Geometry: see drawing. Coordinates: mm, zero at the bounding-box minimum. A direction names the side the tool comes from. Give positions to 0.01 mm unless a question says otherwise; leave off trailing zeros. Loops run counter-clockwise (first coordinate to the right, second up) from the corner with the lowest first, then second, coordinate; pieces in that order, holes last. Notation, with made-up numbers: M -20.5,88.25 L -10.5,88.25 A16 ccw -10.5,113.25 Z; hole C 30,57 d5. An arc over 180 degrees is marked long. Put each result on its own line as item: value.
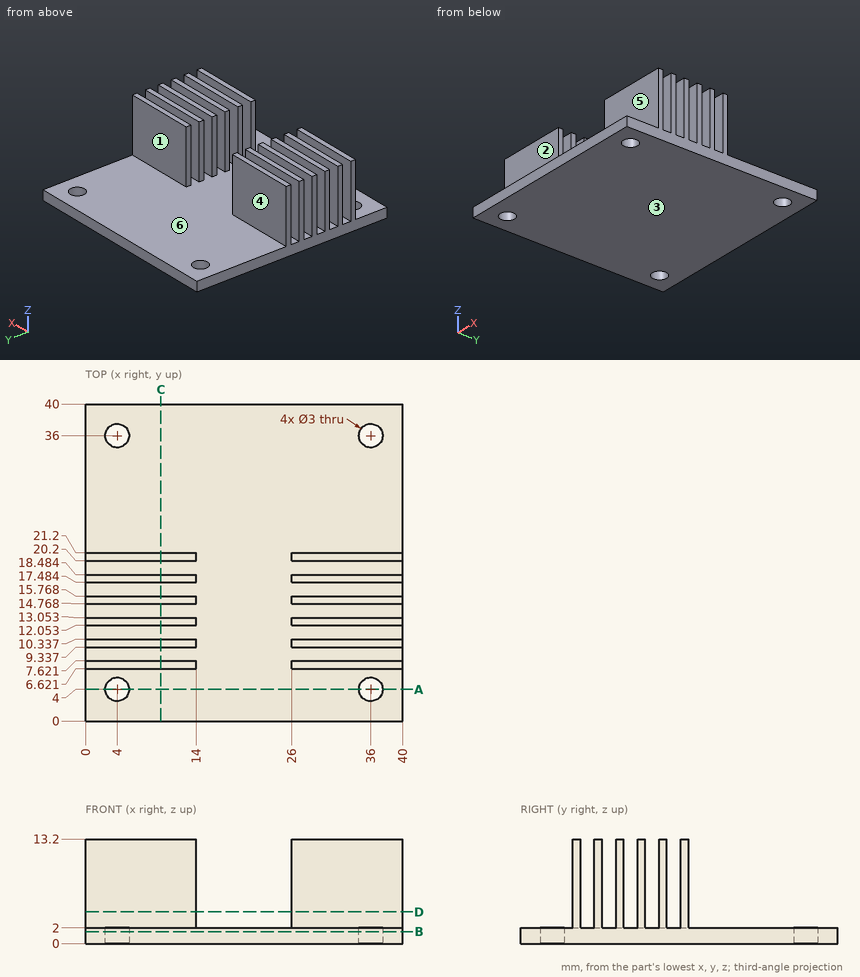
Item 1: Line query: probe 1 along Y at (x, z) = (7.5, 3.25) (1 decimal); probe 2 along Y at (x, z) = (36, 1.55); probe 3 along X at (y, z) = (12.5, 11.75). Output: solid intervals per line, ascending. Write a range as [from, to].
Output values:
probe 1: [6.6, 7.6], [9.3, 10.3], [12.1, 13.1], [14.8, 15.8], [17.5, 18.5], [20.2, 21.2]
probe 2: [0, 2.5], [5.5, 34.5], [37.5, 40]
probe 3: [0, 14], [26, 40]
Item 2: Section B-B on z = 1.5. Output: boundary loops of the cut face in (x, y).
Output values:
outline: M 0,0 L 40,0 L 40,40 L 0,40 Z; hole C 4,4 d3; hole C 4,36 d3; hole C 36,4 d3; hole C 36,36 d3
Item 3: Set-up query: the marked faces 1, 2 and 3. Return all of +Z, -Z, +X, -X, +Y, -Y with unobstructed straight access to the full face (end or side cutting, diameter ignored); none if empty.
Output values:
face 1: +Z, +X, -X, +Y
face 2: +Z, +X, -X, -Y
face 3: -Z, +X, -X, +Y, -Y
Item 4: Section A-A on y = 4. Output: boundary loops of the cut face in (x, z).
Output values:
outline: M 0,0 L 2.5,0 L 2.5,2 L 0,2 Z; M 5.5,0 L 34.5,0 L 34.5,2 L 5.5,2 Z; M 37.5,0 L 40,0 L 40,2 L 37.5,2 Z
Item 5: Section D-D on z = 4. Count the separate pieces of the cut face and the enclosed holes in it, then the cut area to 3 significant figures.
Output values:
separate pieces: 12
enclosed holes: 0
area: 168 mm²
Item 6: Pin query (flat end, axial travel): pin 1 Ø5.5 at (x, z) = (30.5, 10.5) entering from +Y; pin 2 Ø5.5 at (x, z) = (34.5, 9) entering from -Y; pin 3 Ø2.5 at (x, y) = (36, 36) entering from -Z; pin 4 Ø2 at (x, y) = (29, 32.5) entering from +Z. Return the tip coordinate at first contact, or that it passes through.
Output values:
pin 1: y = 21.2
pin 2: y = 6.62
pin 3: through
pin 4: z = 2
Item 7: Section C-C on x = 9.5. Output: boundary loops of the cut face in (y, z) (1 decimal).
Output values:
outline: M 0,0 L 40,0 L 40,2 L 21.2,2 L 21.2,13.2 L 20.2,13.2 L 20.2,2 L 18.5,2 L 18.5,13.2 L 17.5,13.2 L 17.5,2 L 15.8,2 L 15.8,13.2 L 14.8,13.2 L 14.8,2 L 13.1,2 L 13.1,13.2 L 12.1,13.2 L 12.1,2 L 10.3,2 L 10.3,13.2 L 9.3,13.2 L 9.3,2 L 7.6,2 L 7.6,13.2 L 6.6,13.2 L 6.6,2 L 0,2 Z
Item 8: Mould query, pull axis Y, two halves, no side actions, for the marked faces 4, 5 and 6. Classes: pulls with the +Y half, pulls with the -Y half, needs draft (parallel to the pull), parting line crosses it, or undercut.
Output values:
face 4: pulls with the +Y half
face 5: pulls with the -Y half
face 6: undercut
